Geometry: final body of the model. Coordinates: model frame, mm. A direction names the side the tool comes from. Give positions to 0.01 mm unless a question says otherwise; leave off trailing zeros. Order: outer loops, then holes, each group sorted by start corner. A loop starts at its lowest first (then second) coordinate and runs counter-clockwise, first axis right, second up. Notation, with made-up numbers: (-33.75, 29.25) - (-1.75, 29.25) arc R9 ccw to (-1.75, 45.25) - close; hole circle Ø11 at (-23.5, -39.75). An arc over 180 degrees is marked (long way). One line per question, with ' | ' between items. Start each with the question number.
from build123d import *

# Parameters (mm, degrees)
SKETCH1_W           = 80
SKETCH1_H           = 80
BOSS_EXTRUDE1_DEPTH = 3
SKETCH2_R           = 1.25
CUT_EXTRUDE1_DEPTH  = 3
SKETCH3_R           = 1.25
CUT_EXTRUDE2_DEPTH  = 3
CUT_EXTRUDE3_DEPTH  = 3
SKETCH5_R           = 13.5
CUT_EXTRUDE4_DEPTH  = 3
CUT_EXTRUDE5_DEPTH  = 24


with BuildPart() as part:
    # Sketch1 → Boss-Extrude1 (new body)
    with BuildSketch(Plane.XY):
        with Locations((40, 40)):
            Rectangle(SKETCH1_W, SKETCH1_H)
    extrude(amount=BOSS_EXTRUDE1_DEPTH)

    # Sketch2 → Cut-Extrude1 (cut)
    with BuildSketch(Plane.XY.offset(3)):
        with Locations((3, 77)):
            Circle(SKETCH2_R)
    extrude(amount=-CUT_EXTRUDE1_DEPTH, mode=Mode.SUBTRACT)

    # Sketch3 → Cut-Extrude2 (cut)
    with BuildSketch(Plane.XY.offset(3)):
        with Locations((77, 3)):
            Circle(SKETCH3_R)
    extrude(amount=-CUT_EXTRUDE2_DEPTH, mode=Mode.SUBTRACT)

    # Sketch4 → Cut-Extrude3 (cut)
    with BuildSketch(Plane(origin=(0, 3.75760721, 3), x_dir=(1, 0, 0), z_dir=(0, 0, 1))):
        Polygon((40, 34), (56, 34), (56, 50), (56, 66), (40, 66), (24, 66), (24, 34), align=None)
    extrude(amount=-CUT_EXTRUDE3_DEPTH, mode=Mode.SUBTRACT)

    # Sketch5 → Cut-Extrude4 (cut)
    with BuildSketch(Plane(origin=(0, 0.849012918, 3), x_dir=(1, 0, 0), z_dir=(0, 0, 1))):
        with Locations((40, 19.003705046)):
            Circle(SKETCH5_R)
    extrude(amount=-CUT_EXTRUDE4_DEPTH, mode=Mode.SUBTRACT)

    # Sketch6 → Cut-Extrude5 (cut)
    with BuildSketch(Plane.XY.offset(3)):
        Polygon((70, 59), (70, 54), (65, 54), (65, 59), (65, 61), (70, 61), align=None)
    extrude(amount=-CUT_EXTRUDE5_DEPTH, mode=Mode.SUBTRACT)


solid = part.part
(1) Cut plane A-A, the plane y = 52. Return the cut outline in (x, z), plus the area to 3 significant figures.
(2) Pull-direction query (X, two-part tool) for faces 3 (the flat face through (39, 0, 1)), 4 (the flat face through (80, 39, 1)), 5 (the flat face through (68, 54, 2)), 6 (the cylindrical face through (2.84, 78.24, 1.52)); classes: +X half, -X half, draft (parallel to the pull), parting line (faces both ways), or undercut.
(3) Material intervals for line 1 along Y through (x, z) = (3, 0.75); line 2 along Y through (x, z) = (77, 1.6); line 3 along X through (y, z) = (40, 1.15), sorted ascending. Write a range as from..to.
(4) Cut plane B-B, the plane x = 3. Return the cut outline in (y, z), plus the area to 4 significant figures.
(5) Cut plane C-C, the plane x = 38. Return the cut outline in (y, z).
(6) Cut plane D-D, the plane z = 0.8. Return the cut outline in (x, y), plus the area to 3 significant figures.
(7) Contact query for a flat-ended pin moving along its axis: P1, Ø1.5, axis at x = 15, y = 30, coming from the -Z side. Output: stop coordinate, or through.
(8) Access query for faces 1 (the flat face through (31, 32, 3)), 2 (the flat face through (40, 69.758, 2)). Directions: +Z, -Z, +X, -X, +Y, -Y. A direction counts if a zero-diameter tool reaches every point of the face in a straight line with its end or side. Return the directions, or none.
Results are:
1) outline: (0, 0) - (24, 0) - (24, 3) - (0, 3) - close; (56, 0) - (80, 0) - (80, 3) - (56, 3) - close | area: 144 mm2
2) face 3: draft | face 4: +X half | face 5: undercut | face 6: undercut
3) line 1: 0..75.75, 78.25..80 | line 2: 0..1.75, 4.25..80 | line 3: 0..24, 56..80
4) outline: (0, 0) - (75.75, 0) - (75.75, 3) - (0, 3) - close; (78.25, 0) - (80, 0) - (80, 3) - (78.25, 3) - close | area: 232.5 mm2
5) outline: (0, 0) - (6.5, 0) - (6.5, 3) - (0, 3) - close; (33.2, 0) - (37.76, 0) - (37.76, 3) - (33.2, 3) - close; (69.76, 0) - (80, 0) - (80, 3) - (69.76, 3) - close
6) outline: (0, 0) - (80, 0) - (80, 80) - (0, 80) - close; hole circle Ø2.5 at (3, 77); hole (24, 37.76) - (56, 37.76) - (56, 69.76) - (24, 69.76) - close; hole circle Ø27 at (40, 19.85); hole (65, 54) - (70, 54) - (70, 61) - (65, 61) - close; hole circle Ø2.5 at (77, 3) | area: 4,760 mm2
7) P1: z = 0
8) face 1: +Z, +X, -X, +Y, -Y | face 2: +Z, -Z
